Read the model definition and answer for the solid it produces. Units are mm, in the model's axes. Face numbers are marked on the shaded views. A direction names the side the tool comes from. Coordinates: 2 decimals unless noted, no trailing zeros. Loops run counter-clockwise (first coordinate to the right, second up) from the corner with the lowest first, then second, coordinate; pieces in that order, holes last. Notation, with made-up numbers: (-8, -20.5) -> (-2, -20.5) arc R37 cw to (-2, 16.5) -> close; hole circle Ø1 at (24, -5). An arc over 180 degrees is marked (long way). Answer in a Markdown table with one row per item.
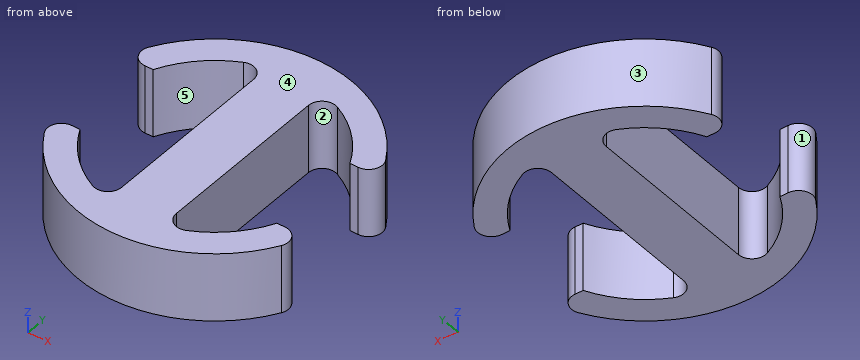
```python
from build123d import *

# Parameters (mm, degrees)
BOSS_EXTRUDE1_DEPTH = 5


with BuildPart() as part:
    # Sketch1 → Boss-Extrude1 (new body)
    with BuildSketch(Plane.XY):
        with BuildLine():
            Line((-2, -6.32455532), (-2, 6.32455532))
            ThreePointArc((-2, 6.32455532), (-2.465477516, 7.169709575), (-3.428571429, 7.228063223))
            ThreePointArc((-3.428571429, 7.228063223), (-5.628767855, 5.684801882), (-7.193747285, 3.5))
            Line((-7.193747285, 3.5), (-7.794228634, 3.5))
            ThreePointArc((-7.794228634, 3.5), (-8.660254038, 4), (-8.660254038, 5))
            ThreePointArc((-8.660254038, 5), (0, 10), (8.660254038, 5))
            ThreePointArc((8.660254038, 5), (8.660254038, 4), (7.794228634, 3.5))
            Line((7.794228634, 3.5), (7.193747285, 3.5))
            ThreePointArc((7.193747285, 3.5), (5.628767855, 5.684801882), (3.428571429, 7.228063223))
            ThreePointArc((3.428571429, 7.228063223), (2.465477516, 7.169709575), (2, 6.32455532))
            Line((2, 6.32455532), (2, -6.32455532))
            ThreePointArc((2, -6.32455532), (2.465477516, -7.169709575), (3.428571429, -7.228063223))
            ThreePointArc((3.428571429, -7.228063223), (5.628767855, -5.684801882), (7.193747285, -3.5))
            Line((7.193747285, -3.5), (7.794228634, -3.5))
            ThreePointArc((7.794228634, -3.5), (8.660254038, -4), (8.660254038, -5))
            ThreePointArc((8.660254038, -5), (0, -10), (-8.660254038, -5))
            ThreePointArc((-8.660254038, -5), (-8.660254038, -4), (-7.794228634, -3.5))
            Line((-7.794228634, -3.5), (-7.193747285, -3.5))
            ThreePointArc((-7.193747285, -3.5), (-5.628767855, -5.684801882), (-3.428571429, -7.228063223))
            ThreePointArc((-3.428571429, -7.228063223), (-2.465477516, -7.169709575), (-2, -6.32455532))
        make_face()
    extrude(amount=BOSS_EXTRUDE1_DEPTH)


solid = part.part
```
1. A cutting plane is placed at C-C on y = 4.5. Give the vertices of the cut face in (x, z), and give its area (3 significant figures).
A:
| item | result |
|---|---|
| outline | (-8.79, 0) -> (-6.61, 0) -> (-6.61, 5) -> (-8.79, 5) -> close; (-2, 0) -> (2, 0) -> (2, 5) -> (-2, 5) -> close; (6.61, 0) -> (8.79, 0) -> (8.79, 5) -> (6.61, 5) -> close |
| area | 41.8 mm2 |
2. A tool of negligible diameter and unlimited length cuts with its end or side. For the marked faces 1 and 2, from which of +Z, -Z, +X, -X, +Y, -Y can it reach the whole face along a straight path? Write none if from no direction.
A:
| item | result |
|---|---|
| face 1 | +Z, -Z, -X |
| face 2 | +Z, -Z |
3. A cutting plane is placed at B-B on z = 1.25. Give the vertices of the cut face in (x, y), and give its area (3 significant figures).
A:
| item | result |
|---|---|
| outline | (-8.66, -5) arc R10 ccw to (8.66, -5) arc R1 ccw to (7.79, -3.5) -> (7.19, -3.5) arc R8 cw to (3.43, -7.23) arc R1 cw to (2, -6.32) -> (2, 6.32) arc R1 cw to (3.43, 7.23) arc R8 cw to (7.19, 3.5) -> (7.79, 3.5) arc R1 ccw to (8.66, 5) arc R10 ccw to (-8.66, 5) arc R1 ccw to (-7.79, 3.5) -> (-7.19, 3.5) arc R8 cw to (-3.43, 7.23) arc R1 cw to (-2, 6.32) -> (-2, -6.32) arc R1 cw to (-3.43, -7.23) arc R8 cw to (-7.19, -3.5) -> (-7.79, -3.5) arc R1 ccw to start |
| area | 147 mm2 |
4. Given pin 1 Ø1 at (y, z) = (6, 3.5) entering from +X; pin 2 Ø2.5 at (y, z) = (3, 2.5) entering from -X; pin 3 Ø0.7 at (x, z) = (7.5, 3.5) entering from +Y, each flat-ended and moving along its own axis, determine where each tip first touches the part or whether it passes through.
A:
| item | result |
|---|---|
| pin 1 | stops at x = 8.35 |
| pin 2 | stops at x = -8.76 |
| pin 3 | stops at y = 6.99 |
5. Find the intervals of material crossed by probe 1 along X at (y, z) = (-4.5, 1.55); probe 2 along X at (y, z) = (-7, 0.8); probe 3 along X at (y, z) = (-0.25, 1.2), in increasing order.
A:
| item | result |
|---|---|
| probe 1 | x = -8.79 to -6.61, -2 to 2, 6.61 to 8.79 |
| probe 2 | x = -7.14 to -3.87, -2.26 to 2.26, 3.87 to 7.14 |
| probe 3 | x = -2 to 2 |
6. A cutting plane is placed at A-A on x = -4. Give the vertices of the cut face in (y, z), and give its area (3 significant figures).
A:
| item | result |
|---|---|
| outline | (-9.17, 0) -> (-6.93, 0) -> (-6.93, 5) -> (-9.17, 5) -> close; (6.93, 0) -> (9.17, 0) -> (9.17, 5) -> (6.93, 5) -> close |
| area | 22.4 mm2 |
7. A cutting plane is placed at D-D on x = 7.5. Give the vertices of the cut face in (y, z).
A:
| item | result |
|---|---|
| outline | (-6.61, 0) -> (-3.5, 0) -> (-3.5, 5) -> (-6.61, 5) -> close; (3.5, 0) -> (6.61, 0) -> (6.61, 5) -> (3.5, 5) -> close |
8. The mould has two halves that part along Y. Classify the marked faces 3, 4 and 5: pulls with the +Y half, pulls with the -Y half, needs draft (parallel to the pull), parting line crosses it, or undercut.
A:
| item | result |
|---|---|
| face 3 | pulls with the +Y half |
| face 4 | needs draft |
| face 5 | undercut |
